The listing builds one solid part. Answer for the finished solid, in the listing's coordinates (mm). Face numbers are marked on the shaded views. A direction names the side the tool comes from. Round coordinates to 2 decimals unless told otherwise and drop trailing zeros. Loops run counter-clockwise (first coordinate to the right, second up) from the corner with the lowest first, then second, coordinate; pieces in that order, holes last. Notation, with made-up numbers: (47.5, 19.25) - (80.5, 19.25) arc R17 ccw to (80.5, 23.25) - close; hole circle Ø6 at (-30, -8). An arc over 180 degrees is marked (long way). One line per item, written item: value.
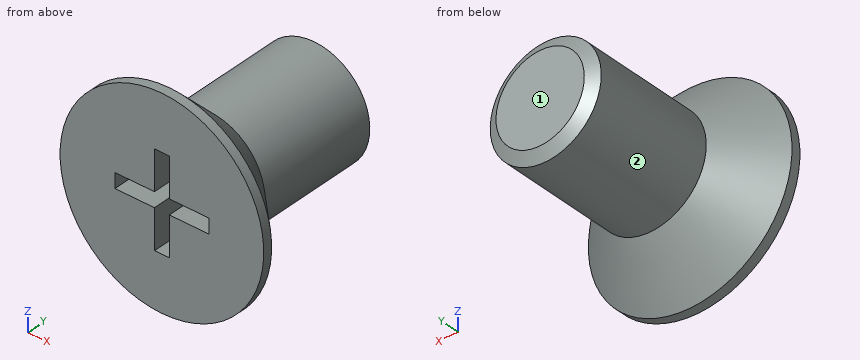
```python
from build123d import *

# Parameters (mm, degrees)
POCKET_DEPTH = 3.81


with BuildPart() as part:
    # Sketch → Revolution (revolve)
    with BuildSketch(Plane.YZ):
        Polygon((0, 0), (0, 5.5), (0.5, 5.5), (3, 3), (9.64493, 3), (10, 2.385), (10, 0), align=None)
    revolve(axis=Axis((0, 0, 0), (0, 1, 0)))

    # Sketch001 → Pocket (cut)
    with BuildSketch(Plane(origin=(0, 0, 0), x_dir=(0, 0, -1), z_dir=(0, -1, 0))):
        Polygon((-2.54, 0.4), (-0.4, 0.4), (-0.4, 2.54), (0.4, 2.54), (0.4, 0.4), (2.54, 0.4), (2.54, -0.4), (0.4, -0.4), (0.4, -2.54), (-0.4, -2.54), (-0.4, -0.4), (-2.54, -0.4), align=None)
    extrude(amount=-POCKET_DEPTH, mode=Mode.SUBTRACT)


solid = part.part
```
1) A cutting plane is placed at B-B on y = 2. Give the vertices of the cut face in (x, z).
Final values:
outline: circle Ø8 at (0, 0); hole (-2.54, -0.4) - (-0.4, -0.4) - (-0.4, -2.54) - (0.4, -2.54) - (0.4, -0.4) - (2.54, -0.4) - (2.54, 0.4) - (0.4, 0.4) - (0.4, 2.54) - (-0.4, 2.54) - (-0.4, 0.4) - (-2.54, 0.4) - close
2) Consider L1, parallel to X at y = 1.5, z = 0.75; L2, parallel to X at y = 1.5, z = -0.5; L3, parallel to Y at x = 4.25, z = -2.25. Determine where each line is inside the solid, lowest interval first.
Final values:
L1: -4.44 to -0.4, 0.4 to 4.44
L2: -4.47 to -0.4, 0.4 to 4.47
L3: 0 to 1.19
3) A cutting plane is placed at A-A on z = 0. Give the vertices of the cut face in (x, y) (3 decimals), and give its area (3 significant figures).
Final values:
outline: (-5.5, 0) - (-2.54, 0) - (-2.54, 3.81) - (2.54, 3.81) - (2.54, 0) - (5.5, 0) - (5.5, 0.5) - (3, 3) - (3, 9.645) - (2.385, 10) - (-2.385, 10) - (-3, 9.645) - (-3, 3) - (-5.5, 0.5) - close
area: 49.2 mm2
4) A cutting plane is placed at D-D on y = 8.75. Give the vertices of the cut face in (x, z), and give its area (3 significant figures).
Final values:
outline: circle Ø6 at (0, 0)
area: 28.3 mm2
5) Each of these flat-tipped pins is pushed along its axis until it touches: pin 1 Ø6 at (x, y) = (-0.5, 8) entering from -Z; pin 2 Ø4 at (x, y) = (0.5, 4.5) entering from +Z; pin 3 Ø1.1 at (x, y) = (2, 3) entering from +Z; pin 4 Ø2 at (x, z) = (-3, -2) entering from -Y. Where does it stop, or does it pass through?
Final values:
pin 1: z = -3
pin 2: z = 3.48
pin 3: z = 3.02
pin 4: y = 0
6) A cutting plane is placed at C-C on x = 0. Give the vertices of the cut face in (y, z) (3 decimals).
Final values:
outline: (0, -5.5) - (0.5, -5.5) - (3, -3) - (9.645, -3) - (10, -2.385) - (10, 2.385) - (9.645, 3) - (3, 3) - (0.5, 5.5) - (0, 5.5) - (0, 2.54) - (3.81, 2.54) - (3.81, -2.54) - (0, -2.54) - close
7) For the marked faces 1 and 2, determine the directions among +Z, -Z, +X, -X, +Y, -Y from which every point of the face is accessible in a straight line to the end or side of a thin tool.
Final values:
face 1: +Z, -Z, +X, -X, +Y
face 2: +Y
